Source: CAD feature listing. Evaluate the final solid. Frame: model axes, mm. Face numbers are marked on the shaded views. A direction names the side the tool comes from. Round coordinates to 2 decimals unless told otherwise and drop trailing zeros. Loops run counter-clockwise (first coordinate to the right, second up) from the corner with the lowest first, then second, coordinate; pieces in that order, holes last. Notation, with made-up numbers: (41, -31.75) - (64, -31.75) arc R20 ccw to (64, -19.75) - close; hole circle Ø11 at (-39.75, -22). An arc over 180 degrees is marked (long way). Use CSV: the item, a comma, the result in double quotes. Start each with the question number.
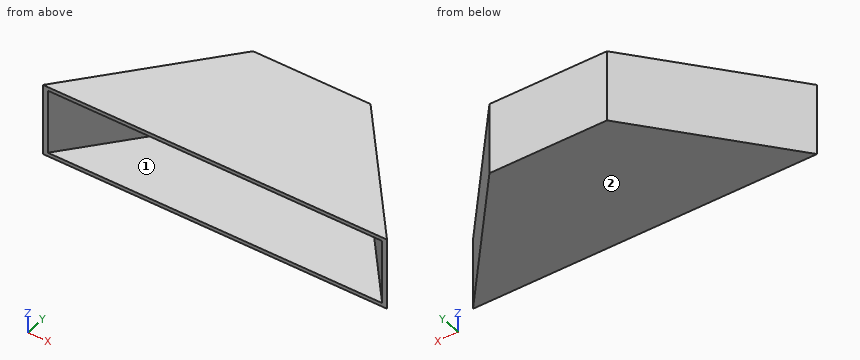
from build123d import *

# Parameters (mm, degrees)
F1_DEPTH = 2
F3_DEPTH = 35
F5_DEPTH = 2


# Not quite as in the source:
# - a feature names something its author has since deleted; it is built from what else it names


with BuildPart() as f1:
    # F0 (on Top) → F1 (new body)
    with BuildSketch(Plane.XY):
        Polygon((-31.75, 72.9657332071), (-92.9755198226, 0), (92.9755198226, 0), (31.75, 72.9657332071), align=None)
    extrude(amount=F1_DEPTH)

    # F2 (on face) → F3 (join)
    with BuildSketch(Plane.XY.offset(2)):
        Polygon((30.8173846837, 70.9657332071), (90.364705244, 0), (92.9755198226, 0), (31.75, 72.9657332071), (-31.75, 72.9657332071), (-92.9755198226, 0), (-90.364705244, 0), (-30.8173846837, 70.9657332071), align=None)
    extrude(amount=F3_DEPTH)

    # F4 (on face) → F5 (join)
    with BuildSketch(Plane.XY.offset(37)):
        Polygon((-31.75, 72.9657332071), (-92.9755198226, 0), (92.9755198226, 0), (31.75, 72.9657332071), align=None)
    extrude(amount=F5_DEPTH)


solid = f1.part
1. Section query D-D on y = 59.5. Return the cut outline in (x, z).
2. Line query: line 1 along Z through (x, y) = (37, 39); line 2 along X through (y, z) = (30, 29); line 3 along X through (y, z) = (66, 23.5). Output: solid intervals per line, ascending.
3. Reachability of the marked faces 1 and 2 from +Z, -Z, +X, -X, +Y, -Y: full face, straight path, thin tool, end or side. Return the list, or none.
4. Contact query for flat-ended pins moving along their axis: P1, Ø12, axis at y = 22.5, z = 12.5, coming from the +X side; P2, Ø12, axis at y = 32.5, z = 27.5, coming from the +X side; P3, Ø8, axis at y = 12, z = 20.5, coming from the -X side. Output: stop coordinate, or through.
5. Section query A-A on x = 6. Return the cut outline in (y, z), and give its area (3 significant figures).
6. Section query B-B on y = 67. Return the cut outline in (x, z).
7. Section query C-C on z = 11. Return the cut outline in (x, y), and give its area (3 significant figures).
Values:
1,outline,"(-43.05, 0) - (43.05, 0) - (43.05, 39) - (-43.05, 39) - close; hole (-40.44, 2) - (40.44, 2) - (40.44, 37) - (-40.44, 37) - close"
2,line 1,"z = 0 to 2, 37 to 39"
2,line 2,"x = -67.8 to -65.19, 65.19 to 67.8"
2,line 3,"x = -37.59 to -34.98, 34.98 to 37.59"
3,face 1,"-Y"
3,face 2,"-Z, +X, -X, +Y, -Y"
4,P1,"stops at x = 79.13"
4,P2,"stops at x = 70.74"
4,P3,"stops at x = -86.26"
5,outline,"(0, 0) - (72.97, 0) - (72.97, 39) - (0, 39) - (0, 37) - (70.97, 37) - (70.97, 2) - (0, 2) - close"
5,area,"362 mm^2"
6,outline,"(-36.76, 0) - (36.76, 0) - (36.76, 39) - (-36.76, 39) - close; hole (-34.15, 2) - (34.15, 2) - (34.15, 37) - (-34.15, 37) - close"
7,outline,"(-92.98, 0) - (-90.36, 0) - (-30.82, 70.97) - (30.82, 70.97) - (90.36, 0) - (92.98, 0) - (31.75, 72.97) - (-31.75, 72.97) - close"
7,area,"501 mm^2"
